from build123d import *

# Parameters (mm, degrees)
F0_W     = 177.8
F0_H     = 63.5
F1_DEPTH = 50.8
F2_W     = 40.907368
F2_H     = 50.8
F3_DEPTH = 25.4
F4_W     = 27.672634
F4_H     = 27.94
F5_DEPTH = 25.4
F6_W     = 13.016606
F6_H     = 27.94
F7_DEPTH = 45.466
F8_W     = 172.72
F8_H     = 58.42
F9_DEPTH = 74.93


with BuildPart() as f1:
    # F0 (on Top) → F1 (new body)
    with BuildSketch(Plane.XY):
        Rectangle(F0_W, F0_H)
    extrude(amount=F1_DEPTH)

    # F2 (on face) → F3 (join)
    with BuildSketch(Plane.XZ.offset(31.75)):
        with Locations((46.772763, 25.4)):
            Rectangle(F2_W, F2_H)
    extrude(amount=F3_DEPTH)

    # F4 (on face) → F5 (cut)
    with BuildSketch(Plane.XZ.offset(57.15)):
        with Locations((46.772763, 13.97)):
            Rectangle(F4_W, F4_H)
    extrude(amount=-F5_DEPTH, mode=Mode.SUBTRACT)

    # F6 (on face) → F7 (cut)
    with BuildSketch(Plane(origin=(26.319079, 0, 0), x_dir=(0, -1, 0), z_dir=(-1, 0, 0))):
        with Locations((44.45, 13.97)):
            Rectangle(F6_W, F6_H)
    extrude(amount=-F7_DEPTH, mode=Mode.SUBTRACT)

    # F8 (on face) → F9 (cut)
    with BuildSketch(Plane(origin=(0, 0, 0), x_dir=(1, 0, 0), z_dir=(0, 0, -1))):
        Rectangle(F8_W, F8_H)
    extrude(amount=-F9_DEPTH, mode=Mode.SUBTRACT)


solid = f1.part
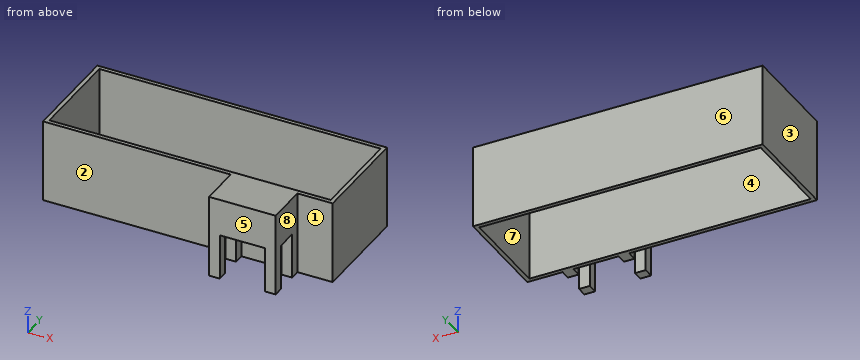
Design review of the part built by this model. Coordinates are the model's own, in mm. Face numbers are marked on the shaded views. A direction names the side the tool comes from. Round coordinates to 2 decimals unless told otherwise and drop trailing zeros. Order: outer loops, then holes, each group sorted by start corner. A loop starts at its lowest first (then second) coordinate and runs counter-clockwise, first axis right, second up. Notation, with made-up numbers: M 53.25,37 L 110.25,37 A23 ccw 110.25,68 Z; hole C 56,82.5 d11. An arc over 180 degrees is marked long. Answer as CSV lines item,"result". Start each with the question number.
1) Wall thickness on line 1 along Y through (x, z) = (63, 44); line 2 along X through (y, z) = (-25, 32.5); line 3 along Y through (x, z) = (-23, 44.5): over which ranges is each line inside the solid? List them lowest first. Write a range as [from, to].
2) Tool access review of the marked faces 1, 2, 3, 4 and 5: name each direction out of +Z, -Z, +X, -X, +Y, -Y from which nothing blocks a thin tool from reaching the whole face with its end or side.
3) Add section C-C (y = 13.5). Give the boundary of the cut face in (x, z), then the cut area to 3 significant figures.
4) Add section D-D (z = 47). Give the boundary of the cut face in (x, y), then the cut area to 3 significant figures.
5) For pin 1 Ø20.5 at (y, z) = (-43.5, 36.5) entering from -X; pin 2 Ø6.5 at (x, z) = (82.5, 15.5) entering from -Y; pin 3 Ø3 at (y, z) = (-34.5, 15.5) entering from +X, all flat-tipped, find the tip position at first contact; note any pin that passes through.
6) Add section B-B (z = 5.5). Give the boundary of the cut face in (x, y), then the cut area to 3 significant figures.
7) Add section A-A (x = 17.5). Give the boundary of the cut face in (y, z), then the cut area to 3 significant figures.
8) The part is to be moulded in two halves that separate along X. For the marked faces 6, 7 and 8, say which applies: +X half, -X half, draft (parallel to the pull), parting line (faces both ways), or undercut.
Resolved:
1,line 1,"[-57.15, -29.21], [29.21, 31.75]"
1,line 2,"[-88.9, -86.36], [86.36, 88.9]"
1,line 3,"[-31.75, -29.21], [29.21, 31.75]"
2,face 1,"+Z, -Z, +X, -Y"
2,face 2,"+Z, -Z, -X, -Y"
2,face 3,"+Z, -Z, -X, +Y, -Y"
2,face 4,"+Z, -Z"
2,face 5,"+Z, -Z, +X, -X, -Y"
3,outline,"M -88.9,0 L -86.36,0 L -86.36,50.8 L -88.9,50.8 Z; M 86.36,0 L 88.9,0 L 88.9,50.8 L 86.36,50.8 Z"
3,area,"258 mm^2"
4,outline,"M -88.9,-31.75 L 26.32,-31.75 L 26.32,-57.15 L 67.23,-57.15 L 67.23,-31.75 L 88.9,-31.75 L 88.9,31.75 L -88.9,31.75 Z; hole M -86.36,-29.21 L 86.36,-29.21 L 86.36,29.21 L -86.36,29.21 Z"
4,area,"2,240 mm^2"
5,pin 1,"x = 26.32"
5,pin 2,"y = -31.75"
5,pin 3,"x = 67.23"
6,outline,"M -88.9,-31.75 L 26.32,-31.75 L 26.32,-37.94 L 32.94,-37.94 L 32.94,-31.75 L 60.61,-31.75 L 60.61,-37.94 L 67.23,-37.94 L 67.23,-31.75 L 88.9,-31.75 L 88.9,31.75 L -88.9,31.75 Z; M 26.32,-57.15 L 32.94,-57.15 L 32.94,-50.96 L 26.32,-50.96 Z; M 60.61,-57.15 L 67.23,-57.15 L 67.23,-50.96 L 60.61,-50.96 Z; hole M -86.36,-29.21 L 86.36,-29.21 L 86.36,29.21 L -86.36,29.21 Z"
6,area,"1,360 mm^2"
7,outline,"M -31.75,0 L -29.21,0 L -29.21,50.8 L -31.75,50.8 Z; M 29.21,0 L 31.75,0 L 31.75,50.8 L 29.21,50.8 Z"
7,area,"258 mm^2"
8,face 6,"draft"
8,face 7,"undercut"
8,face 8,"+X half"
